Check sheet for the modelled part. Datum: model origin and axes. Units: mm. Face numbers are marked on the shaded views. A direction names the side the tool comes from. Round coordinates to 2 decimals unless told otherwise and drop trailing zeros. Order: outer loops, then holes, each group sorted by start corner. A loop starts at its lowest first (then second) coordinate and runs counter-clockwise, first axis right, second up. Notation, with made-up numbers: (55.25, -39.75) -> (81.25, -39.75) arc R28 ccw to (81.25, -9.75) -> close; hole circle Ø9 at (49.5, 31.5). An arc over 180 degrees is marked (long way). Answer in a Markdown table with one row per item.
Autodesk Inventor part; units mm, degrees
ref_plane "YZ Plane" through (0, 0, 0) normal (1, 0, 0) x (0, 1, 0)
ref_plane "XZ Plane" through (0, 0, 0) normal (0, 1, 0) x (-1, 0, 0)
ref_plane "XY Plane" through (0, 0, 0) normal (0, 0, 1) x (1, 0, 0)
sketch "Base Profile" plane through (0, 0, 0) normal (0, 1, 0) x (-1, 0, 0)
  line L0 (0, 0) -> (15, 0)
  line L1 (15, 0) -> (15, -15)
  line L2 (15, -15) -> (0, -15)
  line L3 (0, -15) -> (0, 0)
  line L4 (15, -15) -> (15, 0)
  line L5 (15, -15) -> (0, -15)
  line L6 (0, -15) -> (0, -21.35)
  line L7 (0, -21.35) -> (15, -21.35)
  line L8 (15, -21.35) -> (15, -15)
  dimension "d164" = 15
  dimension "d165" = 15
  dimension "d360" = 6.35
extrude "Stock" add sketch "Base Profile" against normal blind 33
extrude "Extrusion Post" add sketch "Base Profile" along normal blind 15 contours L0 L1 L2 L3
sketch "Front Pattern" plane through (0, -33, -21.35) normal (1, 0, 0) x (0, 0, -1)
  line L0 (-21.35, 0) -> (-21.35, 48)
  line L1 (0, 0) -> (-21.35, 0)
  line L2 (0, 33) -> (0, 0)
  line L3 (-6.35, 33) -> (0, 33)
  line L4 (-6.35, 33) -> (-6.35, 48)
  line L5 (-21.35, 48) -> (-6.35, 48)
  circle A0 centre (-13.85, 40.5) radius 3.175
  line L6 (-6.35, 33) -> (-6.35, 0)
  line L7 (-6.35, 16.5) -> (0, 16.5) construction
  circle A1 centre (-3.175, 29.825) radius 3.175
  circle A2 centre (-3.175, 3.175) radius 3.175
  line L8 (-3.175, 26.65) -> (0, 26.65)
  line L9 (-3.175, 6.35) -> (0, 6.35)
  line L10 (-6.35, 33) -> (0, 33)
  point P0 (-3.175, 16.5)
  point P1 (0, 3.175)
  point P2 (0, 29.825)
  point P3 (-6.35, 3.175)
  point P4 (-6.35, 29.825)
  point P5 (-3.175, 0)
  point P6 (-3.175, 33)
  dimension "d408" = 6.35
  dimension "d361" = 6.35
  dimension "d362" = 7.5
  dimension "d363" = 7.5
hole "Hole24" at (0, 7.5, -7.5) direction (-1, 0, 0) diameter 3.2004 end through all counterbore diameter 6.5024 counterbore depth 2.9972
hole "Hole23" at (0, -3.175, -18.175) at (0, -29.825, -18.175) direction (-1, 0, 0) diameter 3.2004 end through all counterbore diameter 6.35 counterbore depth 3
sketch "Sketch36" plane through (0, 15, 0) normal (0, 1, 0) x (1, 0, 0)
  line L0 (-15, 15) -> (-15, 0)
  line L1 (-15, 0) -> (0, 0)
  line L2 (0, 0) -> (0, 15)
  line L3 (0, 15) -> (-15, 15)
  circle A0 centre (-7.5, 7.5) radius 3.175
  dimension "d385" = 6.35
  dimension "d386" = 7.5
  dimension "d387" = 7.5
hole "Hole25" at (-7.5, 15, -7.5) direction (0, -1, 0) diameter 3.4036 end through all counterbore diameter 6.35 counterbore depth 12.675
sketch "Left Pattern" plane through (-15, -33, 0) normal (0, 0, 1) x (1, 0, 0)
  line L0 (0, 0) -> (0, 48)
  line L1 (15, 0) -> (0, 0)
  line L2 (15, 0) -> (15, 48)
  line L3 (0, 48) -> (15, 48)
  circle A0 centre (7.5, 40.5) radius 1.5
  circle A1 centre (7.5, 7.5) radius 1.5
  dimension "d395" = 3
  dimension "d396" = 7.5
  dimension "d397" = 7.5
  dimension "d398" = 3
  dimension "d399" = 7.5
hole "Hole26" at (-7.5, 7.5, 0) at (-7.5, -25.5, 0) direction (0, 0, -1) diameter 2.459 end up to surface
extrude "Extrusion21" cut sketch "Front Pattern" against normal up to surface (3 mm away) contours L6 A2 L1 | A2 L2 L1 | A2 | L3 A1 L6 | A2 L9 L2 | A1 | L3 L2 A1 | A1 L2 L8
fillet "Fillet4" radius 3.175 2 edges at (-9, 0, -21.35) (-9, -33, -21.35)
equation "\"d164\" = extrusionWidth"
equation "\"d168\" = extrusionOffset"
equation "\"extrusionWidth\" = 15"
equation "\"idlerLength\" = 18"
equation "\"bearingOffsetFromBottom\" = 7.5"
equation "\"extrusionOffset\" = 33"
equation "\"bearingStackHeight\" = 9"
equation "\"bearingSlotLength\" = 5"
equation "\"bearingClearance\" = 13"
equation "\"pinSupportLength\" = 2"
properties part number "A Idler" material "Aluminum 6061"
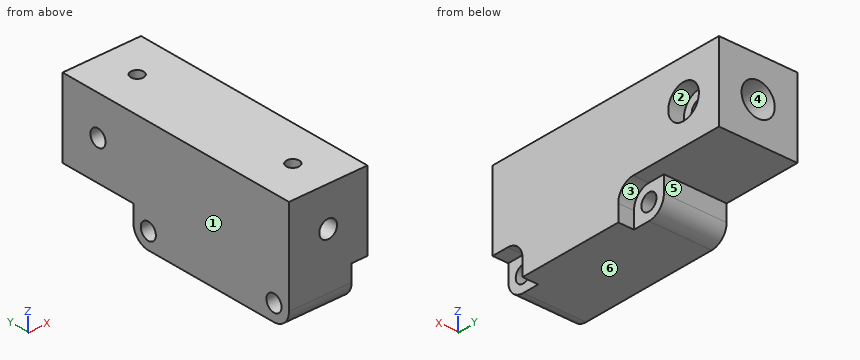
(1) Depth check by flat-ended pin: pin 1 Ø3 at (y, z) = (-31, -17.5) entering from +X; pin 2 Ø3.5 at (x, z) = (-1.5, -20.5) entering from -Y; pin 3 Ø1.5 at (x, z) = (-1.5, -19) entering from +Y. Enter the tip coordinate at first touch or a pass-through.
Solutions:
| item | result |
|---|---|
| pin 1 | x = -3 |
| pin 2 | y = -32.66 |
| pin 3 | y = -6.35 |
(2) Section check A-A on x = -7.5. Give the number of separate pieces and of enclosed holes in the cut face, plus the area to 3 significant figures.
Solutions:
| item | result |
|---|---|
| separate pieces | 4 |
| enclosed holes | 2 |
| area | 684 mm^2 |
(3) Section check D-D on y = -23.5. Record the boundary of the cut face in (x, z), plus the area to 3 significant figures.
Solutions:
| item | result |
|---|---|
| outline | (-15, -21.35) -> (0, -21.35) -> (0, 0) -> (-15, 0) -> close; hole circle Ø3.4 at (-7.5, -7.5) |
| area | 311 mm^2 |
(4) Draft check along Y on the marked faces 1, 2 and 3. Enter one of: pulls with the +Y half, pulls with the -Y half, needs draft (parallel to the pull), parting line crosses it, or undercut.
Solutions:
| item | result |
|---|---|
| face 1 | needs draft |
| face 2 | undercut |
| face 3 | pulls with the +Y half |
(5) Scan lines: probe 1 along Y at (x, z) = (-12.75, -7.5); probe 2 along X at (y, z) = (7.5, -3.5); probe 3 along Z at (x, y) = (-7.5, -15). Record each from-to range of solid material in increasing order. Write a range as from..to.
Solutions:
| item | result |
|---|---|
| probe 1 | -33..5.9, 9.1..15 |
| probe 2 | -15..-8.73, -6.27..0 |
| probe 3 | -21.35..-9.2, -5.8..0 |
(6) Section check B-B on z = -7.5. Record the boundary of the cut face in (x, y) (3 decimals), plus the area to 3 significant figures.
Solutions:
| item | result |
|---|---|
| outline | (-15, -33) -> (-9.202, -33) -> (-9.202, 2.325) -> (-10.675, 2.325) -> (-10.675, 5.9) -> (-15, 5.9) -> close; (-15, 9.1) -> (-10.675, 9.1) -> (-10.675, 15) -> (-15, 15) -> close; (-5.798, -33) -> (0, -33) -> (0, 4.249) -> (-2.997, 4.249) -> (-2.997, 5.9) -> (-4.325, 5.9) -> (-4.325, 2.325) -> (-5.798, 2.325) -> close; (-4.325, 9.1) -> (-2.997, 9.1) -> (-2.997, 10.751) -> (0, 10.751) -> (0, 15) -> (-4.325, 15) -> close |
| area | 482 mm^2 |
(7) Tool access check on the marked faces 4, 5 and 6. Record the directions out of +Z, -Z, +X, -X, +Y, -Y that give a thin tool (end or side, any length) a straight path to the whole face; none if there is none.
Solutions:
| item | result |
|---|---|
| face 4 | +Y |
| face 5 | -Z, +X, -X, +Y |
| face 6 | -Z, +X, -X, +Y, -Y |
